For this review, take the finished solid that the model builds, in its own axes (mm). Give positions to 0.01 mm unless a question says otherwise; leave off trailing zeros. Order: outer loops, then holes, each group sorted by start corner. A loop starts at its lowest first (then second) coordinate and runs counter-clockwise, first axis right, second up.
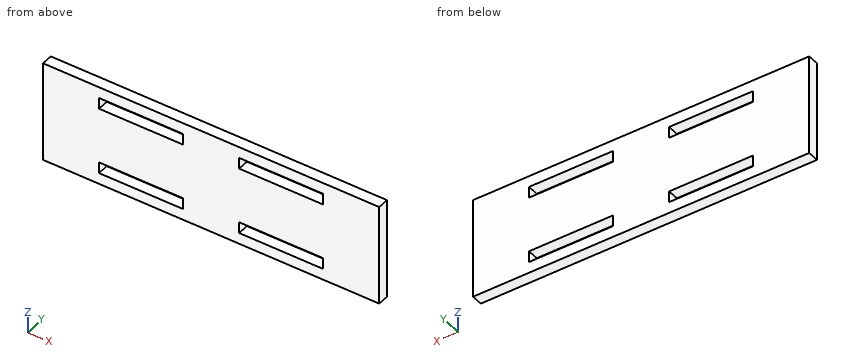
Autodesk Inventor part; units mm, degrees
ref_plane "YZ Plane" through (0, 0, 0) normal (1, 0, 0) x (0, 1, 0)
ref_plane "XZ Plane" through (0, 0, 0) normal (0, 1, 0) x (-1, 0, 0)
ref_plane "XY Plane" through (0, 0, 0) normal (0, 0, 1) x (1, 0, 0)
sketch "Sketch1" plane through (0, 0, 0) normal (0, 1, 0) x (-1, 0, 0)
  line L0 (0, 0) -> (-60, 0)
  line L1 (-60, 0) -> (-60, 18)
  line L2 (-60, 18) -> (0, 18)
  line L3 (0, 18) -> (0, 0)
  dimension "d0" = 60
  dimension "d1" = 18
extrude "Extrusion1" add sketch "Sketch1" along normal blind 2
sketch "Sketch3" plane through (0, 2, 0) normal (0, 1, 0) x (1, 0, 0)
  line L0 (10, -16) -> (25, -16)
  line L1 (25, -16) -> (25, -14)
  line L2 (25, -14) -> (10, -14)
  line L3 (10, -14) -> (10, -16)
  line L4 (10, -2) -> (25, -2)
  line L5 (25, -2) -> (25, -4)
  line L6 (25, -4) -> (10, -4)
  line L7 (10, -4) -> (10, -2)
  line L8 (60, 0) -> (0, 0)
  line L9 (0, 0) -> (0, -18)
  line L10 (0, -18) -> (60, -18)
  line L11 (60, -18) -> (60, 0)
  line L12 (30, 6.382) -> (30, -24.5999) construction
  line L13 (50, -16) -> (35, -16)
  line L14 (35, -16) -> (35, -14)
  line L15 (35, -14) -> (50, -14)
  line L16 (50, -14) -> (50, -16)
  line L17 (50, -2) -> (35, -2)
  line L18 (35, -2) -> (35, -4)
  line L19 (35, -4) -> (50, -4)
  line L20 (50, -4) -> (50, -2)
  dimension "d13" = 15
  dimension "d14" = 2
  dimension "d15" = 15
  dimension "d16" = 2
  dimension "d17" = 10
  dimension "d18" = 0
  dimension "d19" = 2
  dimension "d20" = 10
  dimension "d21" = 10
extrude "Extrusion3" cut sketch "Sketch3" against normal through all contours L3 L2 L1 L0 | L4 L5 L6 L7 | L13 L14 L15 L16 | L20 L19 L18 L17
properties part number "Mounting_base"
1) We need section A-A on x = 47. Give the boundary of the cut face in (y, z), then the cut area to 3 significant figures.
Answer sheet:
outline: (0, 0) - (2, 0) - (2, 2) - (0, 2) - close; (0, 4) - (2, 4) - (2, 14) - (0, 14) - close; (0, 16) - (2, 16) - (2, 18) - (0, 18) - close
area: 28.0 mm2
2) We need section B-B on y = 0.9. Give the boundary of the cut face in (x, z), then the cut area to 3 significant figures.
Answer sheet:
outline: (0, 0) - (60, 0) - (60, 18) - (0, 18) - close; hole (10, 2) - (25, 2) - (25, 4) - (10, 4) - close; hole (10, 14) - (25, 14) - (25, 16) - (10, 16) - close; hole (35, 2) - (50, 2) - (50, 4) - (35, 4) - close; hole (35, 14) - (50, 14) - (50, 16) - (35, 16) - close
area: 960 mm2
3) To check wall thickness, follow line 1 (Z direction, x = 39, y = 0.25); line 2 (X direction, y = 0.15, z = 2.5). State the ranges of each line that lie inside material, in increasing order.
Answer sheet:
line 1: z = 0 to 2, 4 to 14, 16 to 18
line 2: x = 0 to 10, 25 to 35, 50 to 60
4) Clearance check with a flat-ended pin moving along its axis: pin 1 (0.6 mm diameter, centred on y = 0.5, z = 15.5, fed in from -X). State where the tip first meets the part, or that it passes through.
Answer sheet:
pin 1: stops at x = 0
